Work out the finished part from the listing and answer in its coordinate system (mm). Face numbers are marked on the shaded views. A direction names the side the tool comes from. Coordinates: 2 decimals unless noted, no trailing zeros. Loops run counter-clockwise (first coordinate to the right, second up) from the corner with the lowest first, then second, coordinate; pieces in that order, holes last. Notation, with made-up numbers: (42.5, 23.25) - (50.5, 23.25) arc R14 ccw to (50.5, 50.25) - close; hole circle Ø4 at (18, 65). An arc over 180 degrees is marked (long way). Write each question's results on one line, items separated by ' | '. Start each with the question number.
Item 1: Section D-D, the plane z = -1.4 is taken. Write down the section's boundary in (x, y) (3 decimals), plus the area to 3 significant figures.
Item 2: A tool of negligible diameter and unlimited length cuts with its end or side. For the marked faces 3 and 4, from which of +Z, -Z, +X, -X, +Y, -Y can it reach the whole face along a straight path? Write none if from no direction.
Item 3: Section A-A, the plane z = 3.05 is taken. Write down the section's boundary in (x, y) (3 decimals).
Item 4: Section C-C, the plane y = 7.2 is taken. Write down the section's boundary in (x, z), plus the area to 3 significant figures.
Item 5: Consider probe 1 along X at (y, z) = (7.4, 1.6); probe 2 along Y at (x, z) = (10.81, 2.1) (3 decimals); probe 3 along X at (y, z) = (6.6, 1.4). Determine where each line is inside the solid, lowest interval first. Write a range as [from, to].
Item 6: Each of these flat-tipped pins is pushed along its axis until it touches: pin 1 Ø1.5 at (x, y) = (11, 7.5) entering from +Z; pin 2 Ø2.5 at (x, y) = (2, 8) entering from +Z. Where does it stop, or does it pass through?
Item 7: For a pull along X with two mould halves and no side action, classify the marked faces 1 and 2 as +X half, -X half, draft (parallel to the pull), parting line (faces both ways), or undercut.
from build123d import *

# Parameters (mm, degrees)
SKETCH030_R      = 1.5
EXTRUDE031_DEPTH = 4
SKETCH031_R      = 2.5
EXTRUDE030_DEPTH = 4
EXTRUDE037_DEPTH = 2


with BuildPart() as obj1:
    # Sketch030 → Extrude031 (new body)
    with BuildSketch(Plane.XY):
        with Locations((2.15, 7.435)):
            Circle(SKETCH030_R)
        with Locations((10.81, 7.435)):
            Circle(SKETCH030_R)
    extrude(amount=EXTRUDE031_DEPTH)


with BuildPart() as obj2:
    # Sketch031 → Extrude030 (new body)
    with BuildSketch(Plane.XY):
        with Locations((2.15, 7.435)):
            Circle(SKETCH031_R)
        with Locations((10.81, 7.435)):
            Circle(SKETCH031_R)
    extrude(amount=EXTRUDE030_DEPTH)

    # Cut004: cut obj1
    add(obj1.part, mode=Mode.SUBTRACT)


with BuildPart() as obj2_1:
    # Cut004 placement: moved
    add(obj2.part.moved(Location((37, 37.9, 2))))


with BuildPart() as obj2_2:
    # Link005 placement: moved
    add(obj2_1.part.moved(Location((-37, -37.9, -2))))


with BuildPart() as obj3:
    # Sketch037 → Extrude037 (new body)
    with BuildSketch(Plane.XY):
        with BuildLine():
            ThreePointArc((2.15, 9.935), (-0.35, 7.435), (2.15, 4.935))
            Line((2.15, 4.935), (10.81, 4.935))
            ThreePointArc((10.81, 4.935), (13.31, 7.435), (10.81, 9.935))
            Line((10.81, 9.935), (2.15, 9.935))
        make_face()
    extrude(amount=-EXTRUDE037_DEPTH)

    # Fusion010: union obj2
    add(obj2_2.part)


solid = obj3.part
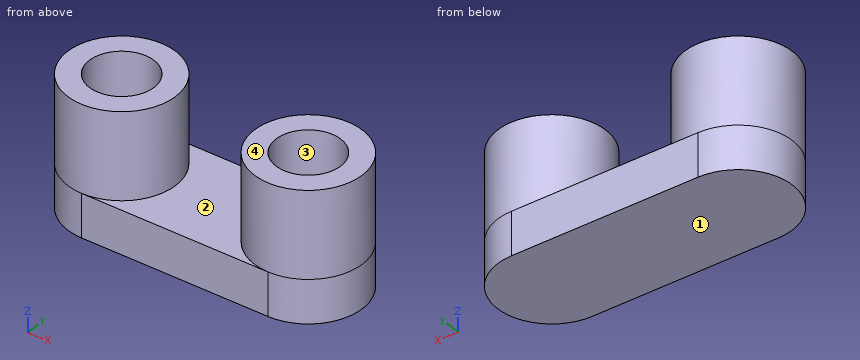
Answer key:
1) outline: (2.15, 4.935) - (10.81, 4.935) arc R2.5 ccw to (10.81, 9.935) - (2.15, 9.935) arc R2.5 ccw to start | area: 62.9 mm^2
2) face 3: +Z | face 4: +Z, +X, -X, +Y, -Y
3) outline: circle Ø5 at (2.15, 7.435); circle Ø5 at (10.81, 7.435); hole circle Ø3 at (2.15, 7.435); hole circle Ø3 at (10.81, 7.435)
4) outline: (-0.34, -2) - (13.3, -2) - (13.3, 4) - (12.29, 4) - (12.29, 0) - (9.33, 0) - (9.33, 4) - (8.32, 4) - (8.32, 0) - (4.64, 0) - (4.64, 4) - (3.63, 4) - (3.63, 0) - (0.67, 0) - (0.67, 4) - (-0.34, 4) - close | area: 43.4 mm^2
5) probe 1: x = [-0.35, 0.65], [3.65, 4.65], [8.31, 9.31], [12.31, 13.31] | probe 2: y = [4.935, 5.935], [8.935, 9.935] | probe 3: x = [-0.21, 0.9], [3.4, 4.51], [8.45, 9.56], [12.06, 13.17]
6) pin 1: stops at z = 0 | pin 2: stops at z = 4
7) face 1: draft | face 2: undercut
